Geometry check sheet. Reference: the model listing, model coordinates, mm. A direction names the side the tool comes from. Give positions to 0.01 mm unless a question says otherwise; leave off trailing zeros. Write each loop counter-clockwise with the first axis right and the second up, starting at its lowest first coordinate (ties: lowest second). Pieces come first, ordered by that corner, then holes. Notation, with made-up numbers: (80.5, 66) -> (115.5, 66) arc R27 ccw to (115.5, 99) -> close; hole circle Ø1 at (55, -6). An arc over 180 degrees is marked (long way). One line per item, written item: value.
from build123d import *

# Parameters (mm, degrees)
SKETCH1_W             = 40
SKETCH1_H             = 30
BOSS_EXTRUDE1_DEPTH   = 10
SKETCH3_R             = 6.625
CUT_EXTRUDE1_DEPTH    = 4.5
SKETCH4_R             = 3.5
CUT_EXTRUDE2_DEPTH    = 27.925824036
F_3_0MM_DOWEL_HOLE1_D = 3
FILLET1_R             = 8.5
SKETCH9_R             = 3.5
CUT_EXTRUDE3_DEPTH    = 5


with BuildPart() as part:
    # Sketch1 → Boss-Extrude1 (new body)
    with BuildSketch(Plane(origin=(0, 0, 0), x_dir=(1, 0, 0), z_dir=(0, 1, 0))):
        Rectangle(SKETCH1_W, SKETCH1_H)
    extrude(amount=BOSS_EXTRUDE1_DEPTH)

    # Sketch3 → Cut-Extrude1 (cut)
    with BuildSketch(Plane.XZ):
        with Locations(Location((0, 0, 0), (0, 0, 270))):
            Circle(SKETCH3_R)
    extrude(amount=-CUT_EXTRUDE1_DEPTH, mode=Mode.SUBTRACT)

    # Sketch4 → Cut-Extrude2 (cut, through all)
    with BuildSketch(Plane(origin=(0, 10, 0), x_dir=(1, 0, 0), z_dir=(0, 1, 0))):
        with Locations(Location((0, 0, 0), (0, 0, 270))):
            Circle(SKETCH4_R)
    extrude(amount=-CUT_EXTRUDE2_DEPTH, mode=Mode.SUBTRACT)

    # Ø3.0mm Dowel Hole1 (through all)
    with Locations(Plane(origin=(0, 10, 0), x_dir=(1, 0, 0), z_dir=(0, 1, 0))):
        with Locations((-14, 9), (-14, -9), (14, -9), (14, 9)):
            Hole(F_3_0MM_DOWEL_HOLE1_D / 2)

    # Fillet1
    fillet1_edges = [part.edges().sort_by_distance(p)[0] for p in [
        (20, 5, 15),
        (-20, 5, 15),
        (-20, 5, -15),
        (20, 5, -15),
    ]]
    fillet(fillet1_edges, radius=FILLET1_R)

    # Sketch9 → Cut-Extrude3 (cut)
    with BuildSketch(Plane(origin=(0, 10, 0), x_dir=(1, 0, 0), z_dir=(0, 1, 0))):
        with Locations(Location((14, -9, 0), (0, 0, 270))):
            Circle(SKETCH9_R)
        with Locations(Location((-14, -9, 0), (0, 0, 270))):
            Circle(SKETCH9_R)
        with Locations(Location((-14, 9, 0), (0, 0, 270))):
            Circle(SKETCH9_R)
        with Locations(Location((14, 9, 0), (0, 0, 270))):
            Circle(SKETCH9_R)
    extrude(amount=-CUT_EXTRUDE3_DEPTH, mode=Mode.SUBTRACT)


solid = part.part
1) Scan lines: probe 1 along X at (y, z) = (3.25, 9); probe 2 along Z at (x, y) = (14, 2.9); probe 3 along Z at (x, y) = (17, 6.5). Record each from-to range of solid material in increasing order.
Verdict:
probe 1: -19.62 to -15.5, -12.5 to 12.5, 15.5 to 19.62
probe 2: -14.62 to -10.5, -7.5 to 7.5, 10.5 to 14.62
probe 3: -12.98 to -10.8, -7.2 to 7.2, 10.8 to 12.98
2) Sectioned sample at B-B on y = 3. Record the cut outline in (x, z) (3 decimals).
Verdict:
outline: (-20, -6.5) arc R8.5 ccw to (-11.5, -15) -> (11.5, -15) arc R8.5 ccw to (20, -6.5) -> (20, 6.5) arc R8.5 ccw to (11.5, 15) -> (-11.5, 15) arc R8.5 ccw to (-20, 6.5) -> close; hole circle Ø3 at (-14, -9); hole circle Ø3 at (-14, 9); hole circle Ø13.25 at (0, 0); hole circle Ø3 at (14, -9); hole circle Ø3 at (14, 9)
3) Sectioned sample at D-D on z = 8. Record the cut outline in (x, y), plus the area to 3 significant figures.
Verdict:
outline: (-19.87, 0) -> (-15.12, 0) -> (-15.12, 5) -> (-17.35, 5) -> (-17.35, 10) -> (-19.87, 10) -> close; (-12.88, 0) -> (12.88, 0) -> (12.88, 5) -> (10.65, 5) -> (10.65, 10) -> (-10.65, 10) -> (-10.65, 5) -> (-12.88, 5) -> close; (15.12, 0) -> (19.87, 0) -> (19.87, 10) -> (17.35, 10) -> (17.35, 5) -> (15.12, 5) -> close
area: 308 mm^2
4) Sectioned sample at C-C on z = 0. Record the cut outline in (x, y) (3 decimals), plus the area to 3 significant figures.
Verdict:
outline: (-20, 0) -> (-6.625, 0) -> (-6.625, 4.5) -> (-3.5, 4.5) -> (-3.5, 10) -> (-20, 10) -> close; (3.5, 4.5) -> (6.625, 4.5) -> (6.625, 0) -> (20, 0) -> (20, 10) -> (3.5, 10) -> close
area: 302 mm^2
5) Mould release check, pull along X, two halves, no side actions. Record for faces 3 (the cylindrical face through (6.57, 2.22, 0.86)), 4 (the flat face through (0, 5, -15)), 5 (the cylindrical face through (17.44, 5.07, 12.58)), 6 (the flat face through (14, 5, 11)): released by +X, released by -X, zero draft, split by the parting line, or undercut.
Verdict:
face 3: undercut
face 4: zero draft
face 5: released by +X
face 6: undercut
6) Sectioned sample at A-A on x = 0. Record the cut outline in (y, z) (3 decimals).
Verdict:
outline: (0, -15) -> (10, -15) -> (10, -3.5) -> (4.5, -3.5) -> (4.5, -6.625) -> (0, -6.625) -> close; (0, 6.625) -> (4.5, 6.625) -> (4.5, 3.5) -> (10, 3.5) -> (10, 15) -> (0, 15) -> close
7) Tool access check on faces 1 (the flat face through (0, 5, 15)), 2 (the cylindrical face through (-16.1, 7.5, 6.2)). Record the directions out of +Z, -Z, +X, -X, +Y, -Y that give a thin tool (end or side, any length) a straight path to the whole face; none if there is none.
Verdict:
face 1: +Z, +X, -X, +Y, -Y
face 2: +Y
8) Depth check by flat-ended pin: pin 1 Ø2 at (y, z) = (1, -9.5) entering from -X; pin 2 Ø2.5 at (x, z) = (-14, 9) entering from +Y; pin 3 Ø6.5 at (x, z) = (1, -2) entering from -Y; pin 4 Ø2 at (x, z) = (-13, 8) entering from +Y. Enter the tip coordinate at first touch or a pass-through.
Verdict:
pin 1: x = -19.76
pin 2: through
pin 3: y = 4.5
pin 4: y = 5
